CAD build for the part. Positions are in the model's coordinates, mm. A direction names the side the tool comes from. Coordinates: 2 decimals unless noted, no trailing zeros. Loops run counter-clockwise (first coordinate to the right, second up) from the corner with the lowest first, then second, coordinate; pieces in that order, holes last.
1) Saw through at C-C, the plane y = -19.5. Write the cut outline in (x, z) (3 decimals), and give its area (3 significant figures).
2) Two-plate mould, pull along Y, no slides. Class faces 4 (the flat face through (73, -30.305, 50)), 5 (the cylindrical face through (-56.22, -13.29, 5.46)), 6 (the flat face through (75.973, -18, 54)): +Y half, -Y half, draft (parallel to the pull), parting line (faces both ways), or undercut.
3) Saw through at A-A, the plane y = -26. Write the cut outline in (x, z), and give its area (3 significant figures).
4) Wall check: line 1 along X through (y, z) = (-25.5, 62.5); line 2 along X through (y, z) = (-15.25, 16.5); line 3 along Y through (x, z) = (-34.5, 51.5). Give the ranges that are in metal, low to high.
5) Pin check, flat tips, straight feed: pin 1 Ø8 at (x, z) = (-3, 25) entering from -Y; pin 2 Ø4 at (x, y) = (29.5, -17) entering from +Z; pin 3 Ø6 at (x, z) = (21.5, 4.5) entering from -Y. Stop position of each tip, or through.
6) Saw through at B-B, the plane z = 89.5. Write the cut outline in (x, y), and give its area (3 significant figures).
7) Which spindle directions (+Z, -Z, +X, -X, +Y, -Y) get a long thin tool onto all of the face, cutting with end or side? Do faces 1 (the flat face through (5, -21.923, 4)), 2 (the flat face through (-68.807, -18, 50)), 3 (the flat face through (-64, -21.923, 55)). Say none if no direction does.
8) Saw through at D-D, the plane x = 49.5. Write the cut outline in (y, z).
```python
from build123d import *

# Parameters (mm, degrees)
F0_W     = 146.05
F0_H     = 25.4
F1_DEPTH = 101.6
F3_DEPTH = 93.98
F5_DEPTH = 101.601
F6_R     = 4.445
F7_DEPTH = 25.401
F8_W     = 1.27
F8_H     = 93.98
F9_DEPTH = 7.62


with BuildPart() as f1:
    # F0 (on Top) → F1 (new body)
    with BuildSketch(Plane.XY):
        with Locations((4.217781, -17.604944)):
            Rectangle(F0_W, F0_H)
    extrude(amount=F1_DEPTH)

    # F2 (on face) → F3 (cut)
    with BuildSketch(Plane.XY.offset(101.6)):
        Polygon((77.242781, -14.302944), (-63.299149, -14.302944), (-68.807219, -14.302944), (-68.807219, -21.922944), (-63.299149, -21.922944), (77.242781, -21.922944), align=None)
    extrude(amount=-F3_DEPTH, mode=Mode.SUBTRACT)

    # F4 (on face) → F5 (cut, through all)
    with BuildSketch(Plane.XY.offset(101.6)):
        Polygon((-61.187219, -21.922944), (-61.187219, -26.113944), (-61.187219, -30.304944), (69.411784, -30.304944), (69.411784, -26.113944), (69.411784, -21.922944), align=None)
    extrude(amount=-F5_DEPTH, mode=Mode.SUBTRACT)

    # F6 (on face) → F7 (cut, through all)
    with BuildSketch(Plane(origin=(0, -4.904944, 0), x_dir=(-1, 0, 0), z_dir=(0, 1, 0))):
        with Locations((-58.192781, 1.016)):
            Circle(F6_R)
        with Locations((56.107219, 1.016)):
            Circle(F6_R)
    extrude(amount=-F7_DEPTH, mode=Mode.SUBTRACT)

    # F8 (on face) → F9 (join)
    with BuildSketch(Plane.XZ.offset(14.302944)):
        with Locations((76.607781, 54.61)):
            Rectangle(F8_W, F8_H)
        with Locations((-68.172219, 54.61)):
            Rectangle(F8_W, F8_H)
    extrude(amount=F9_DEPTH)


solid = f1.part
```
Data:
1. outline: (-68.807, 0) - (-60.435, 0) arc R4.445 cw (long way) to (-51.78, 0) - (53.865, 0) arc R4.445 cw (long way) to (62.52, 0) - (77.243, 0) - (77.243, 101.6) - (75.973, 101.6) - (75.973, 7.62) - (-67.537, 7.62) - (-67.537, 101.6) - (-68.807, 101.6) - close
1. area: 1,270 mm2
2. face 4: -Y half
2. face 5: draft
2. face 6: undercut
3. outline: (-68.81, 0) - (-61.19, 0) - (-61.19, 101.6) - (-68.81, 101.6) - close; (69.41, 0) - (77.24, 0) - (77.24, 101.6) - (69.41, 101.6) - close
3. area: 1,570 mm2
4. line 1: x = -68.81 to -61.19, 69.41 to 77.24
4. line 2: x = -68.81 to -67.54, 75.97 to 77.24
4. line 3: y = -14.3 to -4.9
5. pin 1: stops at y = -14.3
5. pin 2: stops at z = 7.62
5. pin 3: stops at y = -21.92
6. outline: (-68.81, -30.3) - (-61.19, -30.3) - (-61.19, -21.92) - (-67.54, -21.92) - (-67.54, -14.3) - (75.97, -14.3) - (75.97, -21.92) - (69.41, -21.92) - (69.41, -30.3) - (77.24, -30.3) - (77.24, -4.9) - (-68.81, -4.9) - close
6. area: 1,520 mm2
7. face 1: +Z, -Z, -Y
7. face 2: +Z, -Z, -X, +Y, -Y
7. face 3: +Z
8. outline: (-21.92, 0) - (-4.9, 0) - (-4.9, 101.6) - (-14.3, 101.6) - (-14.3, 7.62) - (-21.92, 7.62) - close
